Design review of the part built by this model. Coordinates are the model's own, in mm. A direction names the side the tool comes from. Coordinates: 2 decimals unless noted, no trailing zeros. Order: outer loops, then holes, each group sorted by start corner. A loop starts at its lowest first (then second) coordinate and runs counter-clockwise, first axis right, second up. Notation, with made-up numbers: (-20.75, -1) - (-5.75, -1) arc R12 ccw to (-5.75, 10) - close; hole circle Ø10 at (-20, 8). An arc over 180 degrees is marked (long way). Write each question's results on one line, items separated by ' | '. Start each with the question number.
```python
from build123d import *

# Parameters (mm, degrees)
SKETCH_1_R      = 5
SKETCH_1_R_2    = 1
EXTRUDE_1_DEPTH = 1.5
FILLET_1_R      = 1
SKETCH_2_R      = 2
SKETCH_2_R_2    = 1
EXTRUDE_2_DEPTH = 10


with BuildPart() as part:
    # Эскиз1 → Бобышка-Вытянуть1 (new body)
    with BuildSketch(Plane(origin=(0, 0, 0), x_dir=(1, 0, 0), z_dir=(0, 1, 0))):
        with Locations(Location((0, 0, 0), (0, 0, 270))):
            Circle(SKETCH_1_R)
        with Locations(Location((0, 0, 0), (0, 0, 270))):
            Circle(SKETCH_1_R_2, mode=Mode.SUBTRACT)
    extrude(amount=EXTRUDE_1_DEPTH)

    # Скругление1
    fillet_1_edges = [part.edges().sort_by_distance(p)[0] for p in [
        (0, 1.5, -5),
    ]]
    fillet(fillet_1_edges, radius=FILLET_1_R)

    # Эскиз2 → Бобышка-Вытянуть2 (add)
    with BuildSketch(Plane(origin=(0, 1.5, 0), x_dir=(1, 0, 0), z_dir=(0, 1, 0))):
        with Locations(Location((0, 0, 0), (0, 0, 270))):
            Circle(SKETCH_2_R)
        with Locations(Location((0, 0, 0), (0, 0, 270))):
            Circle(SKETCH_2_R_2, mode=Mode.SUBTRACT)
    extrude(amount=EXTRUDE_2_DEPTH)


solid = part.part
```
(1) Take a section at C-C (y = 1.75). State the section outline as (x, z) points, plus the area to 3 significant figures.
(2) Take a section at A-A (x = 0). State the section outline as (y, z) points, plus the area to 3 significant figures.
(3) To check wall thickness, follow line 1 along X through (y, z) = (9, 0); line 2 along Y through (x, z) = (-2.25, 1); line 3 along Z through (x, y) = (-0.75, 7). State the ranges of each line that lie inside material, in increasing order. Write a range as [from, to].
(4) Take a section at B-B (z = 0). State the section outline as (x, y) points.
(5) Tool access review of faces 1 (the face through (-2, 6, 0)), 2 (the face through (-1, 11.5, 1)): name each direction out of +Z, -Z, +X, -X, +Y, -Y from which nothing blocks a thin tool from reaching the whole face with its end or side.
(6) Mouldability with a two-part tool opening along X and no side actions: class faces 3 (the face through (-1, 6, 0)), 4 (the face through (-4.88, 0.25, -1.08)), 5 (the face through (-1, 1.5, -2)) as +X half, -X half, draft (parallel to the pull), parting line (faces both ways), or undercut.
(7) Clearance check with flat-ended pins moving along their axes: pin 1 (5 mm diameter, centred on x = -0.5, y = 6.5, fed in from +Z); pin 2 (2 mm diameter, centred on x = 1.5, y = 1.5, fed in from +Z); pin 3 (6 mm diameter, centred on x = -2, y = 2, fed in from -Z); pin 4 (3 mm diameter, centred on x = -3, z = 2, fed in from +Y). State where each tip first meets the part, or that it passes through.
Worked out:
1) outline: circle Ø4 at (0, 0); hole circle Ø2 at (0, 0) | area: 9.42 mm^2
2) outline: (0, -5) - (0.5, -5) arc R1 ccw to (1.5, -4) - (1.5, -2) - (11.5, -2) - (11.5, -1) - (0, -1) - close; (0, 1) - (11.5, 1) - (11.5, 2) - (1.5, 2) - (1.5, 4) arc R1 ccw to (0.5, 5) - (0, 5) - close | area: 31.6 mm^2
3) line 1: [-2, -1], [1, 2] | line 2: [0, 1.5] | line 3: [-1.85, -0.66], [0.66, 1.85]
4) outline: (-5, 0) - (-1, 0) - (-1, 11.5) - (-2, 11.5) - (-2, 1.5) - (-4, 1.5) arc R1 ccw to (-5, 0.5) - close; (1, 0) - (5, 0) - (5, 0.5) arc R1 ccw to (4, 1.5) - (2, 1.5) - (2, 11.5) - (1, 11.5) - close
5) face 1: +Y | face 2: +Z, -Z, +X, -X, +Y
6) face 3: undercut | face 4: parting line | face 5: draft
7) pin 1: z = 2 | pin 2: z = 4.9 | pin 3: z = -5 | pin 4: y = 1.5
